For this review, take the finished solid that the model builds, in its own axes (mm). A direction names the side the tool comes from. Coordinates: 2 decimals unless noted, no trailing zeros. Write each loop counter-clockwise with the first axis right and the second up, starting at its lowest first coordinate (ties: lowest second). Pieces come first, ordered by that corner, then holes. Notation, with made-up numbers: (-0.5, -22.75) - (17.5, -22.75) arc R12 cw to (17.5, -6.75) - close; hole circle Ø1 at (31.25, 40.5). An arc over 180 degrees is marked (long way). Use one line per item in the form item = value. Start each with the question number.
1) We need section C-C (x = -15.5). Give the boundary of the cut face in (y, z).
2) Insertion check: P1, Ø1, axis at y = 8, z = 1, coming from the -X side. The pin has a flat end and moves straight along its axis. Give the tip position at first contact, or say it passes through.
3) We need section B-B (y = 50). Give the boundary of the cut face in (x, z), plus the area to 3 significant figures.
4) For L1, parallel to X at y = 26.5, z = 0.55; L2, parallel to X at y = 7, z = 0.8; L3, parallel to Y at x = -3, z = 0.75, list the stretches that pass through material, from the lowest coordinate up. Write a range as from..to.
5) We need section A-A (z = 0.8). Give the boundary of the cut face in (x, y).
6) Mouldability with a two-part tool opening along X and no side actions: class faces 3 (the cylindrical face through (32.06, 26.53, 1.01)), 4 (the flat face through (17, 55, 1)), 5 (the flat face through (12, 48, 1)) as pulls with the +X half, pulls with the -X half, needs draft (parallel to the pull), parting line crosses it, or undercut.
7) We need section D-D (y = 13). Give the boundary of the cut face in (x, z).
8) Tool access review of faces 1 (the cylindrical face through (13.203, 53.859, 1.014)), 2 (the flat face through (0, 28, 0)): name each direction out of +Z, -Z, +X, -X, +Y, -Y from which nothing blocks a thin tool from reaching the whole face with its end or side.
```python
from build123d import *

# Parameters (mm, degrees)
PAD_DEPTH = 2
FILLET_R  = 4


with BuildPart() as part:
    # Sketch → Pad (new body)
    with BuildSketch(Plane.XY):
        Polygon((-22, 0), (22, 0), (22, 19.569513), (25.349717, 16.758767), (33.705955, 26.717345), (22, 36.539808), (22, 55), (12, 55), (12, 44.930804), (0, 55), (-33.705955, 26.717345), (-25.349717, 16.758767), (-22, 19.569513), align=None)
    extrude(amount=PAD_DEPTH)

    # Fillet
    fillet_edges = [part.edges().sort_by_distance(p)[0] for p in [
        (22, 0, 1),
        (25.349717, 16.758767, 1),
        (33.705955, 26.717345, 1),
        (12, 55, 1),
        (22, 55, 1),
        (0, 55, 1),
        (-33.705955, 26.717345, 1),
        (-25.349717, 16.758767, 1),
        (-22, 0, 1),
    ]]
    fillet(fillet_edges, radius=FILLET_R)


solid = part.part
```
Determined:
q1.outline = (0, 0) - (41.99, 0) - (41.99, 2) - (0, 2) - close
q2.P1 = -22
q3.outline = (-5.96, 0) - (5.96, 0) - (5.96, 2) - (-5.96, 2) - close; (12, 0) - (22, 0) - (22, 2) - (12, 2) - close
q3.area = 43.8 mm²
q4.L1 = -32.06..32.06
q4.L2 = -22..22
q4.L3 = 0..52.48
q5.outline = (-31.13, 23.65) - (-27.92, 19.82) arc R4 ccw to (-22.29, 19.33) - (-22, 19.57) - (-22, 4) arc R4 ccw to (-18, 0) - (18, 0) arc R4 ccw to (22, 4) - (22, 19.57) - (22.29, 19.33) arc R4 ccw to (27.92, 19.82) - (31.13, 23.65) arc R4 ccw to (30.64, 29.29) - (22, 36.54) - (22, 51) arc R4 ccw to (18, 55) - (16, 55) arc R4 ccw to (12, 51) - (12, 44.93) - (2.57, 52.84) arc R4 ccw to (-2.57, 52.84) - (-30.64, 29.29) arc R4 ccw to start
q6.face_3 = pulls with the +X half
q6.face_4 = needs draft
q6.face_5 = undercut
q7.outline = (-22, 0) - (22, 0) - (22, 2) - (-22, 2) - close
q8.face_1 = +Z, -Z, +Y
q8.face_2 = -Z, +X, -X, +Y, -Y
